```python
from build123d import *

# Parameters (mm, degrees)
SKETCH1_W           = 28
SKETCH1_H           = 20
BOSS_EXTRUDE1_DEPTH = 3
M3_TAPPED_HOLE1_D   = 2.5
SCALE1_SCALE        = 1.5


with BuildPart() as part:
    # Sketch1 → Boss-Extrude1 (new body)
    with BuildSketch(Plane(origin=(0, 0, 0), x_dir=(1, 0, 0), z_dir=(0, 1, 0))):
        Rectangle(SKETCH1_W, SKETCH1_H)
    extrude(amount=BOSS_EXTRUDE1_DEPTH)

    # M3 Tapped Hole1 (through all)
    with Locations(Plane(origin=(0, 3, 0), x_dir=(1, 0, 0), z_dir=(0, 1, 0))):
        with Locations((-11, 7), (-11, -7), (10, -7), (10, 7)):
            Hole(M3_TAPPED_HOLE1_D / 2)


with BuildPart() as part_1:
    # Scale1: scaled about (0.018168231, 1.5, 0)
    add(part.part.scale(SCALE1_SCALE).moved(Location((-0.009084115, -0.75, 0))))


solid = part_1.part
```
The model under review builds one solid part; all positions refer to its coordinate system, in mm. Coordinates: 2 decimals unless noted, no trailing zeros. Write each loop counter-clockwise with the first axis right and the second up, starting at its lowest first coordinate (ties: lowest second). Pieces come first, ordered by that corner, then holes.
1) We need section A-A on y = 0.95. State the section outline as (x, z) points (3 decimals).
2) We need section B-B on z = -10.5. State the section outline as (x, y) points.
3) To check wall thickness, follow probe 1 along X at (y, z) = (2.5, 10.5); probe 2 along Z at (x, y) = (13.5, 1.4); probe 3 along X at (y, z) = (3.2, 9.75). State the ranges of each line that lie inside material, in increasing order.
4) The part is to be moulded in two halves that separate along Z. For faces 1 (the face through (-16.1, 1.47, 12.33)), 2 (the face through (0, 1, -15)), 3 (the face through (-21.009, 1, 0)), say which applies: pulls with the +Z half, pulls with the -Z half, needs draft (parallel to the pull), parting line crosses it, or undercut.
5) Clearance check with a flat-ended pin moving along its axis: pin 1 Ø5 at (x, z) = (14.99, -10.5) entering from -Y. State where the tip first meets the part, or that it passes through.
6) We need section C-C on x = 16. State the section outline as (y, z) points, then the cut area to 3 significant figures.
Answer list:
1. outline: (-21.009, -15) - (20.991, -15) - (20.991, 15) - (-21.009, 15) - close; hole circle Ø3.75 at (-16.509, -10.5); hole circle Ø3.75 at (-16.509, 10.5); hole circle Ø3.75 at (14.991, -10.5); hole circle Ø3.75 at (14.991, 10.5)
2. outline: (-21.01, -0.75) - (-18.38, -0.75) - (-18.38, 3.75) - (-21.01, 3.75) - close; (-14.63, -0.75) - (13.12, -0.75) - (13.12, 3.75) - (-14.63, 3.75) - close; (16.87, -0.75) - (20.99, -0.75) - (20.99, 3.75) - (16.87, 3.75) - close
3. probe 1: x = -21.01 to -18.38, -14.63 to 13.12, 16.87 to 20.99
3. probe 2: z = -15 to -11.64, -9.36 to 9.36, 11.64 to 15
3. probe 3: x = -21.01 to -18.23, -14.79 to 13.27, 16.71 to 20.99
4. face 1: undercut
4. face 2: pulls with the -Z half
4. face 3: needs draft
5. pin 1: stops at y = -0.75
6. outline: (-0.75, -15) - (3.75, -15) - (3.75, -12.08) - (-0.75, -12.08) - close; (-0.75, -8.92) - (3.75, -8.92) - (3.75, 8.92) - (-0.75, 8.92) - close; (-0.75, 12.08) - (3.75, 12.08) - (3.75, 15) - (-0.75, 15) - close
6. area: 107 mm2
